```python
from build123d import *

# Parameters (mm, degrees)
F0_W            = 50.8
F0_H            = 38.1
F1_DEPTH        = 76.2
F3_DEPTH        = 82.551
F4_D            = 3.6576
F5_D            = 3.5687
F7_D            = 3.7973
F9_D            = 1.9939
F9_DEPTH        = 6.1595
F9_TIP          = 0.5990279941
F11_D           = 2.7051
F11_DEPTH       = 6.35
F11_CBORE_D     = 4.7625
F11_CBORE_DEPTH = 3.81
F11_TIP         = 0.8126940303


with BuildPart() as f1:
    # F0 (on Front) → F1 (new body)
    with BuildSketch(Plane.XZ):
        Polygon((0, 5.4856264032), (0, 0), (88.9, 0), (88.9, 19.05), (82.55, 19.05), (31.75, 19.05), (8.9698585882, 19.05), align=None)
        with Locations((57.15, 38.1)):
            Rectangle(F0_W, F0_H)
    extrude(amount=-F1_DEPTH)

    # F2 (on face) → F3 (cut, through all)
    with BuildSketch(Plane.YZ.offset(82.55)):
        with BuildLine():
            Line((45.72, 57.15), (12.7, 57.15))
            Line((12.7, 57.15), (12.7, 41.402))
            ThreePointArc((12.7, 41.402), (13.4439487758, 39.6059487758), (15.24, 38.862))
            Line((15.24, 38.862), (22.098, 38.862))
            Line((22.098, 38.862), (22.098, 35.052))
            ThreePointArc((22.098, 35.052), (22.8419487758, 33.2559487758), (24.638, 32.512))
            Line((24.638, 32.512), (33.782, 32.512))
            ThreePointArc((33.782, 32.512), (35.5780512242, 33.2559487758), (36.322, 35.052))
            Line((36.322, 35.052), (36.322, 38.862))
            Line((36.322, 38.862), (43.18, 38.862))
            ThreePointArc((43.18, 38.862), (44.9760512242, 39.6059487758), (45.72, 41.402))
            Line((45.72, 41.402), (45.72, 57.15))
        make_face()
    extrude(amount=-F3_DEPTH, mode=Mode.SUBTRACT)

    # F4 (through all)
    with Locations(Plane.YZ.offset(82.55)):
        with Locations((58.674, 52.324), (63.5, 52.324), (63.5, 47.498), (58.674, 47.498)):
            Hole(F4_D / 2)

    # F5 (through all)
    with Locations(Plane.YZ.offset(82.55)):
        with Locations((67.564, 26.924)):
            Hole(F5_D / 2)

    # F7 (through all)
    with Locations(Plane.YZ.offset(88.9)):
        with Locations((67.564, 10.414)):
            Hole(F7_D / 2)

    # F9
    with Locations(Plane.XZ):
        with Locations((47.625, 53.975), (66.675, 53.975), (66.675, 44.45), (47.625, 44.45)):
            Hole(F9_D / 2, depth=F9_DEPTH)
            with Locations((0, 0, -(F9_DEPTH + F9_TIP / 2))):  # 118° drill point
                Cone(0, F9_D / 2, F9_TIP, mode=Mode.SUBTRACT)

    # F11
    with Locations(Plane.XY.offset(57.15)):
        with Locations((41.275, 69.85), (41.275, 52.07), (73.025, 69.85), (73.025, 52.07), (73.025, 6.35), (41.275, 6.35)):
            CounterBoreHole(F11_D / 2, F11_CBORE_D / 2, F11_CBORE_DEPTH, depth=F11_DEPTH)
            with Locations((0, 0, -(F11_DEPTH + F11_TIP / 2))):  # 118° drill point
                Cone(0, F11_D / 2, F11_TIP, mode=Mode.SUBTRACT)


solid = f1.part
```
Model file for the job. Use its own axes, mm. A direction names the side the tool comes from. Coordinates: 2 decimals unless noted, no trailing zeros. Order: outer loops, then holes, each group sorted by start corner. A loop starts at its lowest first (then second) coordinate and runs counter-clockwise, first axis right, second up. Notation, with made-up numbers: (10.25, 44) -> (15.25, 44) arc R13 ccw to (15.25, 57) -> close; hole circle Ø11 at (-40, -20.5). An arc over 180 degrees is marked (long way). Answer as a JSON object with one key per item and string values. Group by question number.
1) Cut at A-A, the plane y = 63.5. Write the cut outline in (x, z).
2) Cut at B-B, the plane y = 41.5. Write the cut outline in (x, z).
3) Drill centre lines: L1, parallel to Y at x = 37, z = 50; L2, parallel to Z at x = 68.5, y = 59; L3, parallel to Z at x = 58, y = 67. Where is each one in solid material? Low to high.
4) Cut at D-D, the plane x = 61. Write the cut outline in (y, z).
5) Pull direction X, two halves, no side cores. Call faces 5 (the face through (82.55, 38, 38)), 6 (the face through (66.65, 6.65, 54.15)), 7 (the face through (58, 40, 38.862)): +X half, -X half, draft (parallel to the pull), parting line (faces both ways), or undercut.
6) Which spindle directions (+Z, -Z, +X, -X, +Y, -Y) get a long thin tool onto all of the face, cutting with end or side? Do faces 1 (the face through (75.296, 52.785, 55.272)), 2 (the face through (48.62, 3.12, 54.02)), 3 (the face through (57.51, 44.96, 39.59)), 4 (the face through (21, 38, 19.05)). Say none if no direction does.
7) Cut at C-C, the plane x = 18. Write the cut outline in (y, z).
8) Flat gauge pins, fed straight in: pin 1 (11.5 mm diameter, centred on y = 35.5, z = 29, fed in from -X); pin 2 (7 mm diameter, centred on x = 87, y = 57, fed in from +Z); pin 3 (2 mm diameter, centred on y = 43, z = 37, fed in from +X). Where does each tip first touch, or does it go through?
Check values:
{
 "1": {"outline": "(0, 0) -> (88.9, 0) -> (88.9, 19.05) -> (82.55, 19.05) -> (82.55, 45.67) -> (31.75, 45.67) -> (31.75, 19.05) -> (8.97, 19.05) -> (0, 5.49) -> close; (31.75, 49.33) -> (82.55, 49.33) -> (82.55, 50.5) -> (31.75, 50.5) -> close; (31.75, 54.15) -> (82.55, 54.15) -> (82.55, 57.15) -> (31.75, 57.15) -> close"},
 "2": {"outline": "(0, 0) -> (88.9, 0) -> (88.9, 19.05) -> (82.55, 19.05) -> (82.55, 38.86) -> (31.75, 38.86) -> (31.75, 19.05) -> (8.97, 19.05) -> (0, 5.49) -> close"},
 "3": {"L1": "y = 0 to 12.7, 45.72 to 76.2", "L2": "z = 0 to 45.7, 49.3 to 50.52, 54.12 to 57.15", "L3": "z = 0 to 8.6, 12.23 to 25.23, 28.62 to 57.15"},
 "4": {"outline": "(0, 0) -> (76.2, 0) -> (76.2, 57.15) -> (45.72, 57.15) -> (45.72, 41.4) arc R2.54 cw to (43.18, 38.86) -> (36.32, 38.86) -> (36.32, 35.05) arc R2.54 cw to (33.78, 32.51) -> (24.64, 32.51) arc R2.54 cw to (22.1, 35.05) -> (22.1, 38.86) -> (15.24, 38.86) arc R2.54 cw to (12.7, 41.4) -> (12.7, 57.15) -> (0, 57.15) -> close; hole circle Ø3.66 at (58.67, 47.5); hole circle Ø3.66 at (58.67, 52.32); hole circle Ø3.66 at (63.5, 47.5); hole circle Ø3.66 at (63.5, 52.32); hole circle Ø3.8 at (67.56, 10.41); hole circle Ø3.57 at (67.56, 26.92)"},
 "5": {"face 5": "+X half", "face 6": "undercut", "face 7": "draft"},
 "6": {"face 1": "+Z", "face 2": "-Y", "face 3": "+Z, +X, -X", "face 4": "+Z, -X, +Y, -Y"},
 "7": {"outline": "(0, 0) -> (76.2, 0) -> (76.2, 19.05) -> (0, 19.05) -> close; hole circle Ø3.8 at (67.56, 10.41)"},
 "8": {"pin 1": "stops at x = 31.75", "pin 2": "stops at z = 19.05", "pin 3": "stops at x = 82.55"}
}
